Read the model definition and answer for the solid it produces. Units are mm, in the model's axes. Face numbers are marked on the shaded views. A direction names the side the tool comes from. Round coordinates to 2 decimals unless told otherwise and drop trailing zeros. Answer as a JSON object with one key per item and string values. Group by question number.
Item 1: Given P1, Ø12, axis at x = 35, z = -11.5, coming from the -Y side; P2, Ø5, axis at x = 34, z = -6.5, coming from the +Y side; P3, Ø4, axis at x = 35, y = 16, coming from the +Z side, each flat-ended and moving along its own axis, determine where each tip first touches the part or whether it passes through.
Item 2: Consider probe 1 along Y at (x, z) = (34.25, 0); probe 2 along Z at (x, y) = (45.25, 7); probe 3 along Y at (x, z) = (34.75, 0). Determine where each line is inside the solid, lowest interval first. Write a range as from..to.
Item 3: The mould has two halves that part along Y. Classify the marked faces 3, 4 and 5: pulls with the +Y half, pulls with the -Y half, needs draft (parallel to the pull), parting line crosses it, or undercut.
Item 4: For the marked faces 1 and 2, determine the directions among +Z, -Z, +X, -X, +Y, -Y from which every point of the face is accessible in a straight line to the end or side of a thin tool.
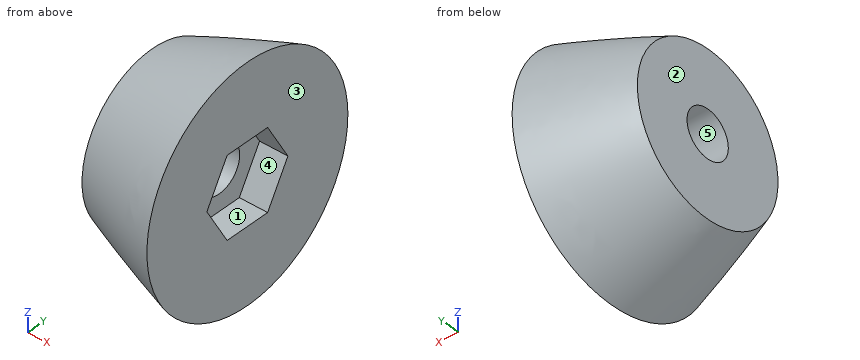
from build123d import *

# Parameters (mm, degrees)
SKIZZE4_R                            = 60
SCHNITT_LINEAR_AUSTRAGEN2_DEPTH      = 30
SKIZZE7_R                            = 100
SCHNITT_LINEAR_AUSTRAGEN4_DEPTH      = 270
SCHNITT_LINEAR_AUSTRAGEN3_DEPTH      = 20
SCHNITT_LINEAR_AUSTRAGEN3_DEPTH_BACK = 6
SKIZZE8_R                            = 5
SCHNITT_LINEAR_AUSTRAGEN5_DEPTH      = 15.138486988


with BuildPart() as part:
    # Skizze2 → Rotation1 (revolve)
    with BuildSketch(Plane.XY):
        with BuildLine():
            add(Edge.make_bspline(
                [(0, 0), (0.001795611, 0.01152954), (0.006532552, 0.034308256), (0.020814366, 0.078703922), (0.056576906, 0.164791889), (0.106248222, 0.260720398), (0.168831035, 0.366307006), (0.257283092, 0.501671411), (0.394318593, 0.693561073), (0.642308836, 1.002302903), (1.094138817, 1.494661034), (1.881119362, 2.241604858), (3.222990514, 3.351501836), (5.484884156, 4.977799832), (9.131242119, 7.255827512), (14.921132384, 10.401183749), (22.887129803, 14.153969102), (35.107137362, 19.201527382), (51.190688574, 24.887218377), (70.271426107, 30.664808891), (92.146031821, 36.297901472), (114.202164386, 41.163847082), (136.396259571, 45.35267271), (158.696515923, 48.929230891), (181.079729625, 51.941229812), (203.527006462, 54.42802234), (226.023091403, 56.423318789), (248.554958993, 57.959192165), (271.111661384, 59.068213328), (291.830400074, 59.728200821), (306.910887079, 60.003248255), (316.347321901, 60.107131137), (320.138486888, 60.138935837)],
                knots=[0, 0, 0, 0, 0, 0.000129466, 0.000258932, 0.000517865, 0.001035729, 0.001329598, 0.001623466, 0.002316092, 0.003657337, 0.005731188, 0.00905026, 0.014374967, 0.023011204, 0.036694212, 0.056839005, 0.087619321, 0.120902055, 0.183694742, 0.246487462, 0.309280168, 0.372072878, 0.43486559, 0.497658301, 0.560451012, 0.623243722, 0.686036437, 0.748829149, 0.811621861, 0.874414574, 0.916582404, 0.916582404, 0.916582404, 0.916582404, 0.916582404], degree=4))
            Line((0, 0), (320.138486888, 0))
            Line((320.138486888, 0), (320.138486888, 60.138935837))
        make_face()
    revolve(axis=Axis((0, 0, 0), (1, 0, 0)))

    # Skizze4 → Schnitt-Linear austragen2 (cut)
    with BuildSketch(Plane(origin=(0, 0, 0), x_dir=(0, 0, -1), z_dir=(1, 0, 0))):
        Circle(SKIZZE4_R)
    extrude(amount=SCHNITT_LINEAR_AUSTRAGEN2_DEPTH, mode=Mode.SUBTRACT)

    # Skizze7 → Schnitt-Linear austragen4 (cut)
    with BuildSketch(Plane(origin=(320.138486888, 0, 0), x_dir=(0, 0, -1), z_dir=(1, 0, 0))):
        Circle(SKIZZE7_R)
    extrude(amount=-SCHNITT_LINEAR_AUSTRAGEN4_DEPTH, mode=Mode.SUBTRACT)

    # Skizze6 → Schnitt-Linear austragen3 (cut, two sides)
    with BuildSketch(Plane(origin=(50.138486888, 0, 0), x_dir=(0, 0, -1), z_dir=(1, 0, 0))) as schnitt_linear_austragen3_sk:
        Polygon((0, -9.814954576), (8.5, -4.907477288), (8.5, 4.907477288), (0, 9.814954576), (-8.5, 4.907477288), (-8.5, -4.907477288), align=None)
    extrude(amount=SCHNITT_LINEAR_AUSTRAGEN3_DEPTH, mode=Mode.SUBTRACT)
    extrude(schnitt_linear_austragen3_sk.sketch, amount=-SCHNITT_LINEAR_AUSTRAGEN3_DEPTH_BACK, mode=Mode.SUBTRACT)

    # Skizze8 → Schnitt-Linear austragen5 (cut, through all)
    with BuildSketch(Plane(origin=(44.138486888, 0, 0), x_dir=(0, 0, -1), z_dir=(1, 0, 0))):
        Circle(SKIZZE8_R)
    extrude(amount=-SCHNITT_LINEAR_AUSTRAGEN5_DEPTH, mode=Mode.SUBTRACT)


solid = part.part
Values found:
{
 "1": {"P1": "y = -19.25", "P2": "y = 18.71", "P3": "z = 13.1"},
 "2": {"probe 1": "-18.7..-5, 5..18.7", "probe 2": "-21.59..-4.88, 4.88..21.59", "probe 3": "-18.89..-5, 5..18.89"},
 "3": {"face 3": "needs draft", "face 4": "undercut", "face 5": "undercut"},
 "4": {"face 1": "+X", "face 2": "+Z, -Z, -X, +Y, -Y"}
}
